Could you check a few things on this drawing? It's one solid part, dimensions in mm from its lowest x, y, z. A direction names the side the tool comes from. Coordinates: 2 decimals unless noted, no trailing zeros. Order: outer loops, then holes, each group sorted by start corner. A loop starts at its lowest first (then second) coordinate and runs counter-clockwise, first axis right, second up. Notation, with made-up numbers: M 21,87 L 27,87 A24 ccw 27,104 Z; hole C 88,46.5 d8. An arc over 180 degrees is marked long. Write item = value, one per line. Start each with the question number.
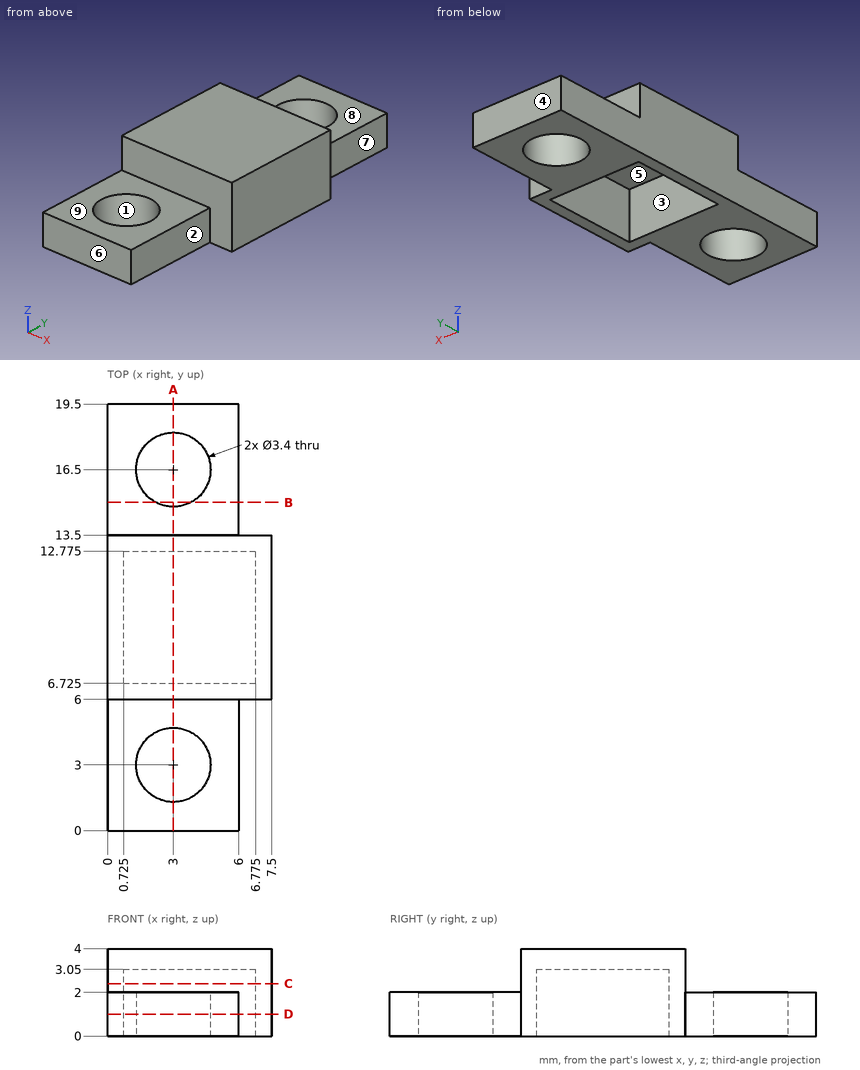
(1) Imagine slicing it at C-C on z = 2.4. List the corners of the cut face in (x, y) for me (3 decimals).
(2) Thinking about a two-plate mould opening in X: for the marked faces 1, 2, 3 and 4, which applies, released by +X, released by -X, zero draft, split by the parting line, or undercut?
(3) Please list where these lines run through material, in increasing order: probe 1 along Y at (x, z) = (3, 0.4) (3 decimals); probe 2 along Y at (x, z) = (2, 2.05) (3 decimals); probe 3 along X at (y, z) = (16.5, 1.3). Write a range as from..to.
(4) Will these pins go through, and if not, where does the flat tip stop? P1, Ø3, axis at x = 4.5, y = 17, coming from the +Z side; P2, Ø1.6, axis at y = 15.5, z = 1, coming from the +X side; P3, Ø3, axis at x = 5, y = 9.5, coming from the -Z side.
(5) Imagine slicing it at B-B on y = 15. List the corners of the cut face in (x, z) for me.
(6) Imagine slicing it at A-A on x = 3. List the corners of the cut face in (y, z) for me (3 decimals), plus the area to 3 significant figures.
(7) Imagine slicing it at D-D on z = 1. List the corners of the cut face in (x, y) for me (3 decimals), plus the area to 3 significant figures.
(8) For the marked faces 5, 6, 7, 8 and 9, which set-ups out of +Z, -Z, +X, -X, +Y, -Y let a thin tool reach every point of the face, with its end or its side?
Response:
q1.outline = M 0,6 L 7.5,6 L 7.5,13.5 L 0,13.5 Z; hole M 0.725,6.725 L 6.775,6.725 L 6.775,12.775 L 0.725,12.775 Z
q2.face_1 = undercut
q2.face_2 = released by +X
q2.face_3 = undercut
q2.face_4 = zero draft
q3.probe_1 = 0..1.3, 4.7..6.725, 12.775..14.8, 18.2..19.5
q3.probe_2 = 6..6.725, 12.775..13.5
q3.probe_3 = 0..1.3, 4.7..6
q4.P1 = 2
q4.P2 = 6
q4.P3 = 3.05
q5.outline = M 0,0 L 2.2,0 L 2.2,2 L 0,2 Z; M 3.8,0 L 6,0 L 6,2 L 3.8,2 Z
q6.outline = M 0,0 L 1.3,0 L 1.3,2 L 0,2 Z; M 4.7,0 L 6.725,0 L 6.725,3.05 L 12.775,3.05 L 12.775,0 L 14.8,0 L 14.8,2 L 13.5,2 L 13.5,4 L 6,4 L 6,2 L 4.7,2 Z; M 18.2,0 L 19.5,0 L 19.5,2 L 18.2,2 Z
q6.area = 21.9 mm2
q7.outline = M 0,0 L 6,0 L 6,6 L 7.5,6 L 7.5,13.5 L 6,13.5 L 6,19.5 L 0,19.5 Z; hole M 0.725,6.725 L 6.775,6.725 L 6.775,12.775 L 0.725,12.775 Z; hole C 3,3 d3.4; hole C 3,16.5 d3.4
q7.area = 73.5 mm2
q8.face_5 = -Z
q8.face_6 = +Z, -Z, +X, -X, -Y
q8.face_7 = +Z, -Z, +X, +Y
q8.face_8 = +Z, +X, -X, +Y
q8.face_9 = +Z, +X, -X, -Y
